Read the model definition and answer for the solid it produces. Units are mm, in the model's axes. Face numbers are marked on the shaded views. A direction names the side the tool comes from. Give positions to 0.01 mm unless a question says otherwise; leave off trailing zeros. Loops run counter-clockwise (first coordinate to the right, second up) from the corner with the lowest first, then second, coordinate; pieces in that order, holes last. Notation, with made-up numbers: (67, -3) - (106, -3) arc R20 ccw to (106, 30) - close; hole circle Ø6 at (12, 1). An arc over 180 degrees is marked (long way). Write item = value, one per line.
```python
from build123d import *

# Parameters (mm, degrees)
BOSS_EXTRUDE1_DEPTH = 4
SKETCH1_3_R         = 2
BOSS_EXTRUDE4_DEPTH = 40
FILLET3_R           = 4
SKETCH4_R           = 3.5
SKETCH4_R_2         = 1.75
BOSS_EXTRUDE5_DEPTH = 6
FILLET2_R           = 4


with BuildPart() as part:
    # Sketch1 → Boss-Extrude1 (new body)
    with BuildSketch(Plane.XY):
        with BuildLine():
            ThreePointArc((16, 10), (14.242640687, 5.757359313), (10, 4))
            Line((10, 4), (140, 4))
            ThreePointArc((140, 4), (135.757359313, 14.242640687), (146, 10))
            Line((146, 10), (146, 100))
            ThreePointArc((146, 100), (135.757359313, 95.757359313), (140, 106))
            Line((140, 106), (10, 106))
            ThreePointArc((10, 106), (14.242640687, 104.242640687), (16, 100))
            ThreePointArc((16, 100), (10, 94), (4, 100))
            Line((4, 100), (4, 10))
            ThreePointArc((4, 10), (10, 16), (16, 10))
        make_face()
    extrude(amount=BOSS_EXTRUDE1_DEPTH)

    # Sketch1<3> → Boss-Extrude4 (add)
    with BuildSketch(Plane.XY):
        with BuildLine():
            ThreePointArc((0, 10), (2.928932188, 2.928932188), (10, 0))
            Line((10, 0), (140, 0))
            ThreePointArc((140, 0), (147.071067812, 2.928932188), (150, 10))
            Line((150, 10), (150, 100))
            ThreePointArc((150, 100), (147.071067812, 107.071067812), (140, 110))
            Line((140, 110), (10, 110))
            ThreePointArc((10, 110), (2.928932188, 107.071067812), (0, 100))
            Line((0, 100), (0, 10))
        make_face()
        with BuildLine():
            Line((140, 4), (10, 4))
            ThreePointArc((10, 4), (14.242640687, 14.242640687), (4, 10))
            Line((4, 10), (4, 100))
            ThreePointArc((4, 100), (14.242640687, 95.757359313), (10, 106))
            Line((10, 106), (140, 106))
            ThreePointArc((140, 106), (135.757359313, 95.757359313), (146, 100))
            Line((146, 100), (146, 10))
            ThreePointArc((146, 10), (135.757359313, 14.242640687), (140, 4))
        make_face(mode=Mode.SUBTRACT)
        with Locations((10, 10)):
            Circle(SKETCH1_3_R, mode=Mode.SUBTRACT)
        with Locations((140, 10)):
            Circle(SKETCH1_3_R, mode=Mode.SUBTRACT)
        with Locations((10, 100)):
            Circle(SKETCH1_3_R, mode=Mode.SUBTRACT)
        with Locations((140, 100)):
            Circle(SKETCH1_3_R, mode=Mode.SUBTRACT)
    extrude(amount=BOSS_EXTRUDE4_DEPTH)

    # Fillet3
    fillet3_edges = [part.edges().sort_by_distance(p)[0] for p in [
        (140, 4, 22),
    ]]
    fillet(fillet3_edges, radius=FILLET3_R)
    fillet3_2_edges = [part.edges().sort_by_distance(p)[0] for p in [
        (4, 100, 22),
        (10, 106, 22),
        (140, 106, 22),
        (146, 100, 22),
        (146, 10, 22),
        (10, 4, 22),
        (4, 10, 22),
    ]]
    fillet(fillet3_2_edges, radius=FILLET3_R)

    # Sketch4 → Boss-Extrude5 (add)
    # profile 1 of 4: a face of its own
    with BuildSketch(Plane.XY.offset(4)):
        with Locations((38, 100)):
            Circle(SKETCH4_R)
        with Locations((38, 100)):
            Circle(SKETCH4_R_2, mode=Mode.SUBTRACT)
    # profile 2 of 4: a face of its own
    with BuildSketch(Plane.XY.offset(4)):
        with Locations((38, 16)):
            Circle(SKETCH4_R)
        with Locations((38, 16)):
            Circle(SKETCH4_R_2, mode=Mode.SUBTRACT)
    # profile 3 of 4: a face of its own
    with BuildSketch(Plane.XY.offset(4)):
        with Locations((125, 16)):
            Circle(SKETCH4_R)
        with Locations((125, 16)):
            Circle(SKETCH4_R_2, mode=Mode.SUBTRACT)
    # profile 4 of 4: a face of its own
    with BuildSketch(Plane.XY.offset(4)):
        with Locations((125, 100)):
            Circle(SKETCH4_R)
        with Locations((125, 100)):
            Circle(SKETCH4_R_2, mode=Mode.SUBTRACT)
    extrude(amount=BOSS_EXTRUDE5_DEPTH)

    # Fillet2
    # the kernel refuses this fillet: 4 mm, written as the material it adds along each edge
    with BuildSketch(Plane(origin=(38, 100, 4), x_dir=(1, 0, 0), z_dir=(0, -1, 0))) as fillet2_piece_1:
        with BuildLine():
            CenterArc((3.5 + FILLET2_R, FILLET2_R), FILLET2_R, 180, 90)
            Line((3.5, FILLET2_R), (3.5, 0))
            Line((3.5, 0), (3.5 + FILLET2_R, 0))
        make_face()
    revolve(axis=Axis((38, 100, 4), (0, 0, 1)))
    with BuildSketch(Plane(origin=(38, 16, 4), x_dir=(1, 0, 0), z_dir=(0, -1, 0))) as fillet2_piece_2:
        with BuildLine():
            CenterArc((3.5 + FILLET2_R, FILLET2_R), FILLET2_R, 180, 90)
            Line((3.5, FILLET2_R), (3.5, 0))
            Line((3.5, 0), (3.5 + FILLET2_R, 0))
        make_face()
    revolve(axis=Axis((38, 16, 4), (0, 0, 1)))
    with BuildSketch(Plane(origin=(125, 16, 4), x_dir=(1, 0, 0), z_dir=(0, -1, 0))) as fillet2_piece_3:
        with BuildLine():
            CenterArc((3.5 + FILLET2_R, FILLET2_R), FILLET2_R, 180, 90)
            Line((3.5, FILLET2_R), (3.5, 0))
            Line((3.5, 0), (3.5 + FILLET2_R, 0))
        make_face()
    revolve(axis=Axis((125, 16, 4), (0, 0, 1)))
    with BuildSketch(Plane(origin=(125, 100, 4), x_dir=(1, 0, 0), z_dir=(0, -1, 0))) as fillet2_piece_4:
        with BuildLine():
            CenterArc((3.5 + FILLET2_R, FILLET2_R), FILLET2_R, 180, 90)
            Line((3.5, FILLET2_R), (3.5, 0))
            Line((3.5, 0), (3.5 + FILLET2_R, 0))
        make_face()
    revolve(axis=Axis((125, 100, 4), (0, 0, 1)))


solid = part.part
```
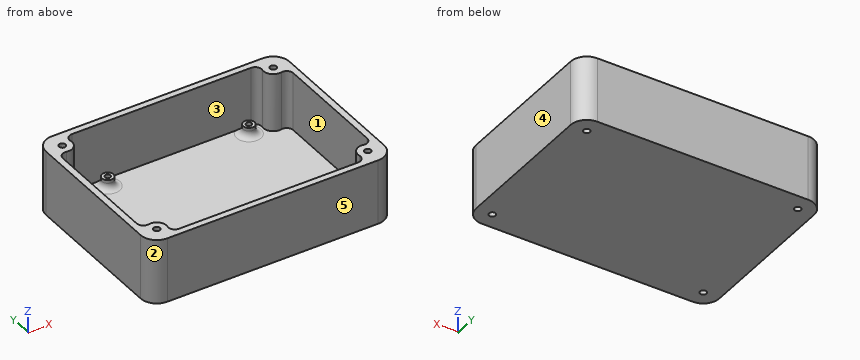
1) A cutting plane is placed at B-B on y = 71. Determine the outline of the cut face in (x, z), then the cut area to 3 significant figures.
Output:
outline = (0, 0) - (150, 0) - (150, 40) - (146, 40) - (146, 4) - (4, 4) - (4, 40) - (0, 40) - close
area = 888 mm²
2) A cutting plane is placed at C-C on z = 24. Determine the outline of the cut face in (x, y), then the cut area to 3 significant figures.
Output:
outline = (0, 10) arc R10 ccw to (10, 0) - (140, 0) arc R10 ccw to (150, 10) - (150, 100) arc R10 ccw to (140, 110) - (10, 110) arc R10 ccw to (0, 100) - close; hole (4, 19.8) arc R4 ccw to (8.8, 15.88) arc R6 cw to (15.88, 8.8) arc R4 ccw to (19.8, 4) - (130.2, 4) arc R4 ccw to (134.12, 8.8) arc R6 cw to (141.2, 15.88) arc R4 ccw to (146, 19.8) - (146, 90.2) arc R4 ccw to (141.2, 94.12) arc R6 cw to (134.12, 101.2) arc R4 ccw to (130.2, 106) - (19.8, 106) arc R4 ccw to (15.88, 101.2) arc R6 cw to (8.8, 94.12) arc R4 ccw to (4, 90.2) - close; hole circle Ø4 at (10, 10); hole circle Ø4 at (10, 100); hole circle Ø4 at (140, 10); hole circle Ø4 at (140, 100)
area = 2,440 mm²
3) The mould has two halves that part along Y. Classify the marked faces 3, 4 and 5: pulls with the +Y half, pulls with the -Y half, needs draft (parallel to the pull), parting line crosses it, or undercut.
Output:
face_3 = undercut
face_4 = needs draft
face_5 = pulls with the -Y half
4) Find the intervals of material crossed by probe 1 along Y at (x, z) = (98, 7.5); probe 2 along Y at (x, z) = (10, 24); probe 3 along X at (y, z) = (34, 19.5), in increasing order.
Output:
probe_1 = 0 to 4, 106 to 110
probe_2 = 0 to 8, 12 to 16, 94 to 98, 102 to 110
probe_3 = 0 to 4, 146 to 150
5) A tool of negligible diameter and unlimited length cuts with its end or side. For the marked faces 1 and 2, from which of +Z, -Z, +X, -X, +Y, -Y can it reach the whole face along a straight path? Write none if from no direction.
Output:
face_1 = +Z
face_2 = +Z, -Z, -X, -Y
6) A cutting plane is placed at A-A on x = 85.5. Determine the outline of the cut face in (y, z), then the cut area to 3 significant figures.
Output:
outline = (0, 0) - (110, 0) - (110, 40) - (106, 40) - (106, 4) - (4, 4) - (4, 40) - (0, 40) - close
area = 728 mm²
7) A cutting plane is placed at D-D on x = 38. Determine the outline of the cut face in (y, z).
Output:
outline = (0, 0) - (110, 0) - (110, 40) - (106, 40) - (106, 4.29) arc R4 cw to (103.5, 8) - (103.5, 10) - (101.75, 10) - (101.75, 4) - (98.25, 4) - (98.25, 10) - (96.5, 10) - (96.5, 8) arc R4 cw to (92.5, 4) - (23.5, 4) arc R4 cw to (19.5, 8) - (19.5, 10) - (17.75, 10) - (17.75, 4) - (14.25, 4) - (14.25, 10) - (12.5, 10) - (12.5, 8) arc R4 cw to (8.5, 4) - (4, 4) - (4, 40) - (0, 40) - close
8) Each of these flat-tipped pins is pushed along its axis until it touches: P1, Ø1, axis at x = 126, y = 100, coming from the +Z side; P2, Ø4, axis at x = 125, y = 15.5, coming from the +Z side. Where does it stop, or does it pass through?
Output:
P1 = 4
P2 = 10
